Check sheet for the modelled part. Datum: model origin and axes. Units: mm. Face numbers are marked on the shaded views. A direction names the side the tool comes from. Give positions to 0.01 mm unless a question says otherwise; leave off trailing zeros. Order: outer loops, then holes, each group sorted by start corner. A loop starts at its lowest first (then second) coordinate and runs counter-clockwise, first axis right, second up. Notation, with made-up numbers: (19, 5) -> (76, 5) arc R14 ccw to (76, 17) -> close; hole circle Ø7 at (-21.5, 55.25). An arc over 180 degrees is marked (long way). Write each question's results on one line, items separated by ' | '.
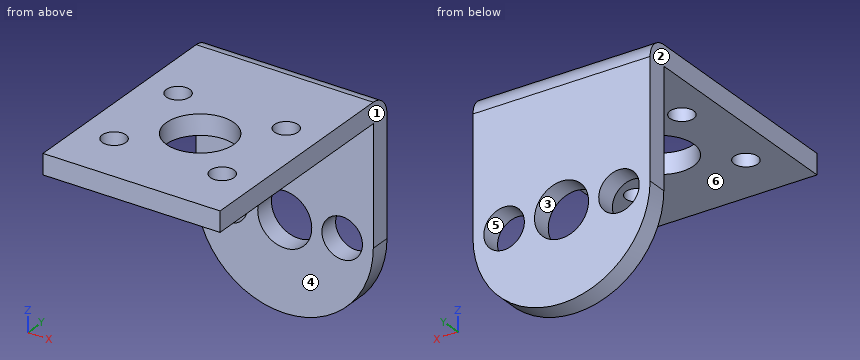
from build123d import *

# Parameters (mm, degrees)
SKETCH_3_R          = 4
EXTRUDE_1_DEPTH     = 3
SKETCH_4_W          = 26.2
SKETCH_4_H          = 33.5
SKETCH_4_R          = 5
SKETCH_4_R_2        = 1.75
EXTRUDE_2_DEPTH     = 3
FILLET_1_R          = 3
SKETCH_7_R          = 3
CUT_EXTRUDE_1_DEPTH = 52.245585176


with BuildPart() as part:
    # 草图3 → 凸台-拉伸1 (new body)
    with BuildSketch(Plane(origin=(0, 0, 0), x_dir=(1, 0, 0), z_dir=(0, 1, 0))):
        with BuildLine():
            Line((0, 0), (-13.1, 0))
            Line((-13.1, 0), (-13.1, 20.4))
            ThreePointArc((-13.1, 20.4), (0, 33.5), (13.1, 20.4))
            Line((13.1, 20.4), (13.1, 0))
            Line((13.1, 0), (0, 0))
        make_face()
        with Locations(Location((0, 20.4, 0), (0, 0, 270))):
            Circle(SKETCH_3_R, mode=Mode.SUBTRACT)
    extrude(amount=-EXTRUDE_1_DEPTH)

    # 草图4 → 凸台-拉伸2 (add)
    with BuildSketch(Plane.XY):
        with Locations((0, -19.75)):
            Rectangle(SKETCH_4_W, SKETCH_4_H)
        with Locations((0, -21.5)):
            Circle(SKETCH_4_R, mode=Mode.SUBTRACT)
        with Locations((8, -28.5)):
            Circle(SKETCH_4_R_2, mode=Mode.SUBTRACT)
        with Locations((8, -14.5)):
            Circle(SKETCH_4_R_2, mode=Mode.SUBTRACT)
        with Locations(Location((-8, -14.5, 0), (0, 0, 180))):
            Circle(SKETCH_4_R_2, mode=Mode.SUBTRACT)
        with Locations(Location((-8, -28.5, 0), (0, 0, 180))):
            Circle(SKETCH_4_R_2, mode=Mode.SUBTRACT)
    extrude(amount=-EXTRUDE_2_DEPTH)

    # 圆角1
    fillet_1_edges = [part.edges().sort_by_distance(p)[0] for p in [
        (0, 0, 0),
    ]]
    fillet(fillet_1_edges, radius=FILLET_1_R)

    # 草图7 → 切除-拉伸1 (cut, through all)
    with BuildSketch(Plane(origin=(0, 0, 0), x_dir=(1, 0, 0), z_dir=(0, 1, 0))):
        with Locations(Location((8.5, 20.4, 0), (0, 0, 270))):
            Circle(SKETCH_7_R)
    cut_extrude_1 = extrude(amount=-CUT_EXTRUDE_1_DEPTH, mode=Mode.SUBTRACT)

    # 镜向1: 切除-拉伸1 across plane
    add(cut_extrude_1.mirror(Plane(origin=(0, 0, 0), x_dir=(0, 0, 1), z_dir=(1, 0, 0))), mode=Mode.SUBTRACT)


solid = part.part
1. Section check B-B on x = 0. Record the cut outline in (y, z), then the cut area to 3 significant figures.
Verdict:
outline: (-36.5, -3) -> (-26.5, -3) -> (-26.5, 0) -> (-36.5, 0) -> close; (-16.5, -3) -> (-3, -3) -> (-3, -16.4) -> (0, -16.4) -> (0, -3) arc R3 ccw to (-3, 0) -> (-16.5, 0) -> close; (-3, -33.5) -> (0, -33.5) -> (0, -24.4) -> (-3, -24.4) -> close | area: 145 mm^2
2. Material ranges on probe 1 along Y at (x, z) = (8, -2.05); probe 2 along X at (y, z) = (-14, -1); probe 3 along Z at (x, y) = (-1.25, -9.5), recorded low to high. Write a range as from..to.
Verdict:
probe 1: y = -36.5..-30.25, -26.75..-16.25, -12.75..-0.15 | probe 2: x = -13.1..-9.68, -6.32..6.32, 9.68..13.1 | probe 3: z = -3..0
3. Gauge pin test, flat ends, axial feed: pin 1 Ø8 at (x, y) = (2, -16.5) entering from -Z; pin 2 Ø4 at (x, z) = (-7.5, -25.5) entering from -Y. Record the tip position at first contact, or that the pin passes through.
Verdict:
pin 1: stops at z = -3 | pin 2: stops at y = -3
4. Access from +Z, -Z, +X, -X, +Y, -Y to the whole of each face (thin tool, end or side, straight path). Record for the marked faces 5 and 6.
Verdict:
face 5: +Y, -Y | face 6: -Z, +X, -X, -Y
5. Mould release check, pull along X, two halves, no side actions. Record for the marked faces 1, 2, 3 and 4: +X half, -X half, draft (parallel to the pull), parting line (faces both ways), or undercut.
Verdict:
face 1: +X half | face 2: -X half | face 3: undercut | face 4: draft
6. Section check C-C on y = -28.5. Record the cut outline in (x, z), then the cut area to 3 significant figures.
Verdict:
outline: (-13.1, -3) -> (-9.75, -3) -> (-9.75, 0) -> (-13.1, 0) -> close; (-6.25, -3) -> (6.25, -3) -> (6.25, 0) -> (-6.25, 0) -> close; (9.75, -3) -> (13.1, -3) -> (13.1, 0) -> (9.75, 0) -> close | area: 57.6 mm^2
7. Section check D-D on x = -8. Record the cut outline in (y, z).
Verdict:
outline: (-36.5, -3) -> (-30.25, -3) -> (-30.25, 0) -> (-36.5, 0) -> close; (-26.75, -3) -> (-16.25, -3) -> (-16.25, 0) -> (-26.75, 0) -> close; (-12.75, -3) -> (-3, -3) -> (-3, -17.44) -> (0, -17.44) -> (0, -3) arc R3 ccw to (-3, 0) -> (-12.75, 0) -> close; (-3, -30.77) -> (0, -30.77) -> (0, -23.36) -> (-3, -23.36) -> close
8. Section check A-A on y = -24.5. Record the cut outline in (x, z).
Verdict:
outline: (-13.1, -3) -> (-4, -3) -> (-4, 0) -> (-13.1, 0) -> close; (4, -3) -> (13.1, -3) -> (13.1, 0) -> (4, 0) -> close
